Design review of the part built by this model. Coordinates are the model's own, in mm. Round coordinates to 2 decimals unless told otherwise and drop trailing zeros. Loops run counter-clockwise (first coordinate to the right, second up) from the corner with the lowest first, then second, coordinate; pieces in that order, holes last. Notation, with made-up numbers: (57, 81) - (98, 81) arc R17 cw to (98, 110) - close; hole circle Ø3 at (35.25, 87). An arc over 180 degrees is marked (long way). Use one line per item in the form item = value. Start each with the question number.
(1) We need section B-B, the plane y = -9. Write out the cut boundary in (x, z).
(2) We need section C-C, the plane y = 7. Write out the cut boundary in (x, z).
(3) We need section A-A, the plane z = 1.1. Write out the cut boundary in (x, y).
(4) For pin 1 (1 mm diameter, centred on y = -3.5, z = 3.5, fed in from +X); pin 2 (1 mm diameter, centred on y = 7, z = 1, fed in from -X), all flat-tipped, find the tip position at first contact; note any pin that passes through.
(5) The part is to be moulded in two halves that separate along Y. For faces 1 (the flat face through (51, 0, 0)), 2 (the cylindrical face through (97.615, 0.751, 2.465)), 3 (the flat face through (51, -15, 2)), say which applies: released by +Y, released by -Y, zero draft, split by the parting line, or undercut.
(6) Wall thickness on probe 1 along Y at (x, z) = (0, 3.8); probe 2 along Y at (x, z) = (-2, 2.85); probe 3 along X at (y, z) = (-7.5, 2.45): over which ranges is each line inside the solid? List them lowest first. Write a range as [from, to].
from build123d import *

# Parameters (mm, degrees)
EXTRUDE_1_DEPTH     = 5
SKETCH_2_R          = 2.5
CUT_EXTRUDE_1_DEPTH = 117.081867662


with BuildPart() as part:
    # 草图1 → 凸台-拉伸1 (new body)
    with BuildSketch(Plane.XY):
        with BuildLine():
            Line((0, 15), (100, 15))
            ThreePointArc((100, 15), (115, 0), (100, -15))
            Line((100, -15), (0, -15))
            ThreePointArc((0, -15), (-15, 0), (0, 15))
        make_face()
    extrude(amount=EXTRUDE_1_DEPTH)

    # 草图2 → 切除-拉伸1 (cut, through all)
    with BuildSketch(Plane(origin=(0, 0, 0), x_dir=(-1, 0, 0), z_dir=(0, 0, -1))):
        Circle(SKETCH_2_R)
        with Locations((-100, 0)):
            Circle(SKETCH_2_R)
    extrude(amount=-CUT_EXTRUDE_1_DEPTH, mode=Mode.SUBTRACT)


solid = part.part
Data:
q1.outline = (-12, 0) - (112, 0) - (112, 5) - (-12, 5) - close
q2.outline = (-13.27, 0) - (113.27, 0) - (113.27, 5) - (-13.27, 5) - close
q3.outline = (0, -15) - (100, -15) arc R15 ccw to (100, 15) - (0, 15) arc R15 ccw to start; hole circle Ø5 at (0, 0); hole circle Ø5 at (100, 0)
q4.pin_1 = 114.7
q4.pin_2 = -13.52
q5.face_1 = zero draft
q5.face_2 = undercut
q5.face_3 = released by -Y
q6.probe_1 = [-15, -2.5], [2.5, 15]
q6.probe_2 = [-14.87, -1.5], [1.5, 14.87]
q6.probe_3 = [-12.99, 112.99]
